```python
from build123d import *

# Parameters (mm, degrees)
SKETCH1_W = 8
SKETCH1_H = 50


with BuildPart() as part:
    # Sketch1 → Revolve1 (revolve)
    with BuildSketch(Plane.XY, mode=Mode.PRIVATE) as revolve1_sk:
        Polygon((35, 18), (0, 18), (0, 15), (38, 15), align=None)
        Polygon((38, 15), (0, 15), (0, 0), (17.5, 0), (38, 0), align=None)
        Polygon((17.5, 0), (0, 0), (0, -44), (8, -44), (17.5, -44), align=None)
        with Locations((4, -69)):
            Rectangle(SKETCH1_W, SKETCH1_H)
        with BuildLine():
            ThreePointArc((8, -94), (5.656854249, -99.656854249), (0, -102))
            Line((0, -102), (0, -94))
            Line((0, -94), (8, -94))
        make_face()
    revolve(revolve1_sk.sketch.rotate(Axis((0, 67.717923126, 0), (0, -1, 0)), 90), axis=Axis((0, 67.717923126, 0), (0, -1, 0)))


solid = part.part
```
Design review of the part built by this model. Coordinates are the model's own, in mm. A direction names the side the tool comes from. Coordinates: 2 decimals unless noted, no trailing zeros. Write each loop counter-clockwise with the first axis right and the second up, starting at its lowest first coordinate (ties: lowest second). Pieces come first, ordered by that corner, then holes.
1) Add section B-B (z = 0). Write out the cut boundary in (x, y).
2) To check wall thickness, follow L1, parallel to Y at x = -26.5, z = -15.5; L2, parallel to Z at x = 32, y = 12; L3, parallel to Z at x = 2, y = -34.5. State the ranges of each line that lie inside material, in increasing order.
3) Add section A-A (x = 0). Write out the cut boundary in (y, z), plus the area to 3 significant figures.
4) Insertion check: pin 1 (1 mm diameter, centred on x = 21.5, z = 28, fed in from +Y); pin 2 (5 mm diameter, centred on x = 5, y = -86, fed in from -Z); pin 3 (12 mm diameter, centred on x = 0.5, y = -12.5, fed in from +Z); pin 4 (4 mm diameter, centred on y = -87.5, z = -2, fed in from +X). Each pin has a flat end and moves straight along its axis. Give the tip position at first contact, or say it passes through.
5) Add section D-D (y = -25.5). Write out the cut boundary in (x, z).
6) Machinability: for faces 1 (the conical face through (34.31, 17.854, -7.619)), 2 (the flat face through (4, -44, -8)), which of the approach directions +Z, -Z, +X, -X, +Y, -Y give a long, thin tool a straight path to every point of the face, cutting with its end or side? Answer none if there is none.
7) Add section C-C (y = -88.5). Write out the cut boundary in (x, z), plus the area to 3 significant figures.
Check result:
1. outline: (-38, 0) - (-17.5, 0) - (-17.5, -44) - (-8, -44) - (-8, -94) arc R8 ccw to (8, -94) - (8, -44) - (17.5, -44) - (17.5, 0) - (38, 0) - (38, 15) - (35, 18) - (-35, 18) - (-38, 15) - close
2. L1: y = 0 to 18
2. L2: z = -20.49 to 20.49
2. L3: z = -17.39 to 17.39
3. outline: (-94, -8) - (-44, -8) - (-44, -17.5) - (0, -17.5) - (0, -38) - (15, -38) - (18, -35) - (18, 35) - (15, 38) - (0, 38) - (0, 17.5) - (-44, 17.5) - (-44, 8) - (-94, 8) arc R8 ccw to start
3. area: 3,800 mm2
4. pin 1: stops at y = 18
4. pin 2: stops at z = -7.6
4. pin 3: stops at z = 17.5
4. pin 4: stops at x = 8
5. outline: circle Ø35 at (0, 0)
6. face 1: +Y
6. face 2: -Y
7. outline: circle Ø16 at (0, 0)
7. area: 201 mm2
